The model under review builds one solid part; all positions refer to its coordinate system, in mm. A direction names the side the tool comes from. Round coordinates to 2 decimals unless told otherwise and drop trailing zeros. Order: outer loops, then holes, each group sorted by start corner. A loop starts at its lowest first (then second) coordinate and runs counter-clockwise, first axis right, second up. Notation, with made-up numbers: (-8, 50) - (49, 50) arc R17 cw to (49, 81) - close; hole circle Ø11 at (74, 78). An arc over 180 degrees is marked (long way). One line per question, with ' | ' between items. Start each with the question number.
Item 1: Add section B-B on x = 0. State the section outline as (y, z) points, and give its area (3 significant figures).
Item 2: Add section C-C on z = 236.25. State the section outline as (x, y) points.
Item 3: Tool access review of faces 1 (the face through (0.222, 0.485, 227.368)), 2 (the face through (0.1, 0.3, 233.6)): name each direction out of +Z, -Z, +X, -X, +Y, -Y from which nothing blocks a thin tool from reaching the whole face with its end or side.
Item 4: Add section A-A on y = 1.4. State the section outline as (x, z) points, and give its area (3 significant figures).
Item 5: For L1, parallel to Y at x = -6.5, z = 236.5; L2, parallel to X at y = 1.4, z = 237.5; L3, parallel to Z at x = 1, y = -0.65, list the stretches that pass through material, from the lowest coordinate up. Write a range as [from, to].
Item 6: Insertion check: pin 1 Ø10 at (x, z) = (-12.5, 228.5) entering from -Y; pin 2 Ø1 at (x, y) = (-0.5, 0.5) entering from -Z. Each pin has a flat end and moves straight along its axis. Give the tip position at first contact, or say it passes through.
Item 7: Add section D-D on z = 231.25. State the section outline as (x, y) points, and give its area (3 significant figures).
from build123d import *

# Parameters (mm, degrees)
SKETCH2_R           = 2.65
BOSS_EXTRUDE1_DEPTH = 2
BOSS_EXTRUDE2_DEPTH = 2
CHAMFER1_SIZE       = 4.5
CHAMFER1_SIZE2      = 0.956504528
BOSS_EXTRUDE3_START = 1
BOSS_EXTRUDE3_DEPTH = 1


with BuildPart() as part:
    # Sketch2 → Boss-Extrude1 (new body)
    with BuildSketch(Plane(origin=(0, 0, 0), x_dir=(1, 0, 0), z_dir=(0, 1, 0))):
        with BuildLine():
            Line((-15.984695958, -228.591802117), (-17.334483725, -247.89466649))
            ThreePointArc((-17.334483725, -247.89466649), (0, -248.5), (17.334483725, -247.89466649))
            Line((17.334483725, -247.89466649), (15.984695958, -228.591802117))
            ThreePointArc((15.984695958, -228.591802117), (0, -229.15), (-15.984695958, -228.591802117))
        make_face()
        with Locations(Location((0, -236.25, 0), (0, 0, 270))):
            Circle(SKETCH2_R, mode=Mode.SUBTRACT)
    extrude(amount=BOSS_EXTRUDE1_DEPTH)

    # Sketch3 → Boss-Extrude2 (add)
    with BuildSketch(Plane(origin=(0, 0, 0), x_dir=(1, 0, 0), z_dir=(0, 1, 0))):
        with BuildLine():
            Line((-15.705670063, -224.601545916), (-15.984695958, -228.591802117))
            ThreePointArc((-15.984695958, -228.591802117), (0, -229.15), (15.984695958, -228.591802117))
            Line((15.984695958, -228.591802117), (15.705670063, -224.601545916))
            ThreePointArc((15.705670063, -224.601545916), (0, -225.15), (-15.705670063, -224.601545916))
        make_face()
    extrude(amount=BOSS_EXTRUDE2_DEPTH)

    # Chamfer1
    chamfer1_edges = [part.edges().sort_by_distance(p)[0] for p in [
        (0, 0, 225.15),
    ]]
    chamfer1_side = [part.faces().sort_by_distance(p)[0] for p in [
        (16.100023839, 0, 236.277479174),
    ]]
    chamfer(chamfer1_edges, length=CHAMFER1_SIZE, length2=CHAMFER1_SIZE2, reference=chamfer1_side[0])

    # Sketch4 → Boss-Extrude3 (add)
    with BuildSketch(Plane.XZ.offset(BOSS_EXTRUDE3_START)):
        with BuildLine():
            Line((-17.334483725, 247.89466649), (-17.038018712, 243.655019276))
            ThreePointArc((-17.038018712, 243.655019276), (0, 244.25), (17.038018712, 243.655019276))
            Line((17.038018712, 243.655019276), (17.334483725, 247.89466649))
            ThreePointArc((17.334483725, 247.89466649), (0, 248.5), (-17.334483725, 247.89466649))
        make_face()
    extrude(amount=-BOSS_EXTRUDE3_DEPTH)

    # Sketch20 → CSK for M3.5 Flat Head Machine Screw2 (revolve, cut)
    with BuildSketch(Plane(origin=(0, 2, 236.25), x_dir=(0, 0, 1), z_dir=(1, 0, 0))):
        Polygon((0, 0), (0, 3), (1.85, 3), (1.85, 2.25), (4.1, 0), align=None)
    revolve(axis=Axis((0, 8.35, 236.25), (0, -1, 0)), mode=Mode.SUBTRACT)


solid = part.part
Determined:
1) outline: (-1, 244.25) - (0, 244.25) - (0, 238.9) - (0.55, 238.9) - (2, 240.35) - (2, 248.5) - (-1, 248.5) - close; (0, 229.65) - (0.96, 225.15) - (2, 225.15) - (2, 232.15) - (0.55, 233.6) - (0, 233.6) - close | area: 36.1 mm2
2) outline: (-16.52, 0) - (-2.65, 0) - (-2.65, 0.55) - (-4.1, 2) - (-16.52, 2) - close; (2.65, 0) - (16.52, 0) - (16.52, 2) - (4.1, 2) - (2.65, 0.55) - close
3) face 1: -Z, -Y | face 2: +Y, -Y
4) outline: (-17.33, 247.89) - (-15.71, 224.6) arc R225.15 cw to (15.71, 224.6) - (17.33, 247.89) arc R248.5 ccw to start; hole circle Ø7 at (0, 236.25) | area: 734 mm2
5) L1: [0, 2] | L2: [-16.61, -3.27], [3.27, 16.61] | L3: [244.25, 248.5]
6) pin 1: y = 0 | pin 2: z = 225.15
7) outline: (-16.17, 0) - (16.17, 0) - (16.17, 2) - (-16.17, 2) - close | area: 64.7 mm2
